Answer from the drawing. Dimensions are ordinates in mm from the lowest x, y and z of the part. A direction names the side the tool comes from. Round coordinates to 2 decimals unless told otherwise and drop trailing zeros. Loops run counter-clockwise (first coordinate to the right, second up) from the corner with the lowest first, then second, coordinate; pieces in that order, holes last. Notation, with made-up numbers: (86, 32.25) - (136, 32.25) arc R20 ccw to (136, 42.25) - close; hole circle Ø8 at (34.5, 70.5). An arc over 180 degrees is marked (long way). Write item = value, one per line. Start each with the question number.
1) A tool of negligible diameter and unlimited length cuts with its end or side. For the marked faces 4 and 5, from which of +Z, -Z, +X, -X, +Y, -Y can it reach the whole face along a straight path? Write none if from no direction.
2) Straight lines are drawn through the part: line 1 along X through (y, z) = (4, 5); line 2 along Y through (x, z) = (43, 18.75); line 3 along X through (y, z) = (6, 18). For each, find the intervals that lie inside material, in ascending order.
3) Section D-D, the plane y = 9.25 is taken. Determine the outline of the cut face in (x, z), and give its area (3 significant figures).
4) For a pull along X with two mould halves and no side action, classify the marked faces 1, 2 and 3 as released by +X, released by -X, zero draft, split by the parting line, or undercut.
5) Section B-B, the plane z = 15 is taken. Determine the outline of the cut face in (x, y), and give its area (3 significant figures).
6) Section C-C, the plane x = 23 is taken. Determine the outline of the cut face in (y, z), and give its area (3 significant figures).
7) Given pin 1 Ø2.5 at (x, z) = (44, 8) entering from -Y; pin 2 Ø4.5 at (y, z) = (7.5, 10) entering from -X; pin 3 Ø1.5 at (y, z) = (6.5, 17.5) entering from +X; pin 4 Ø8 at (x, y) = (14.5, 16) entering from -Z, each flat-ended and moving along its own axis, determine where each tip first touches the part or whether it passes through.
8) Section A-A, the plane y = 13.75 is taken. Determine the outline of the cut face in (x, z).
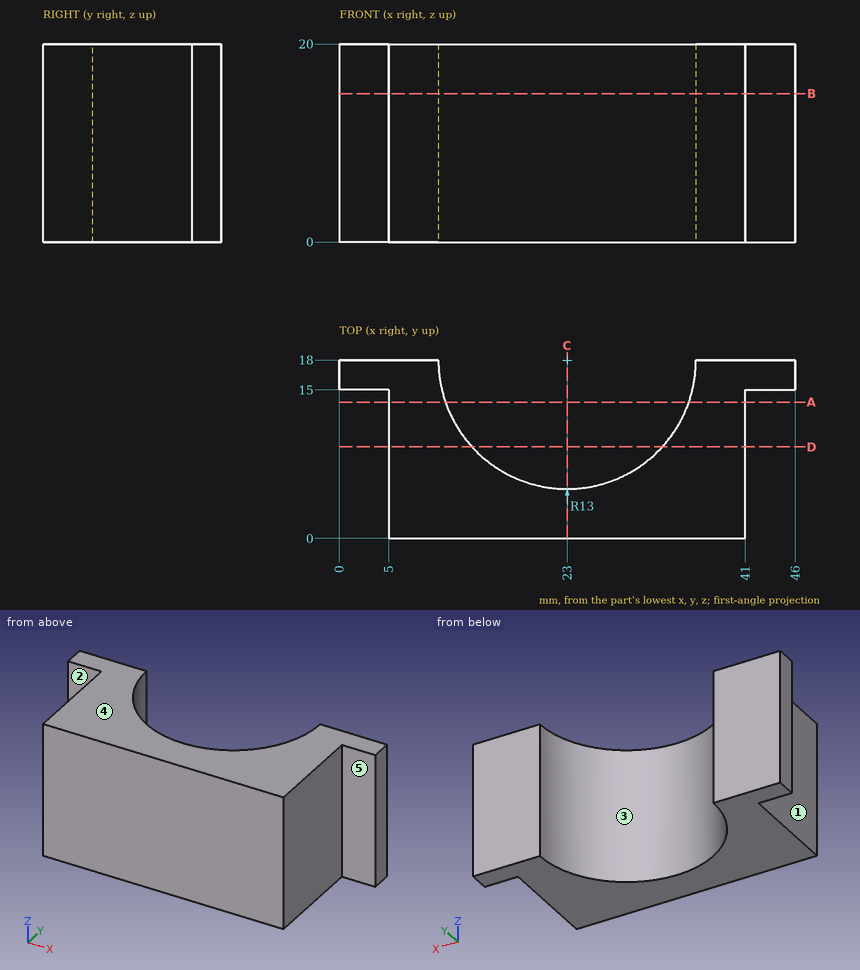
Geometry check:
q1.face_4 = +Z, +X, -X, +Y, -Y
q1.face_5 = +Z, -Z, +X, -Y
q2.line_1 = 5 to 41
q2.line_2 = 15 to 18
q2.line_3 = 5 to 18, 28 to 41
q3.outline = (5, 0) - (13.39, 0) - (13.39, 20) - (5, 20) - close; (32.61, 0) - (41, 0) - (41, 20) - (32.61, 20) - close
q3.area = 335 mm2
q4.face_1 = released by -X
q4.face_2 = zero draft
q4.face_3 = undercut
q5.outline = (0, 15) - (5, 15) - (5, 0) - (41, 0) - (41, 15) - (46, 15) - (46, 18) - (36, 18) arc R13 cw to (10, 18) - (0, 18) - close
q5.area = 413 mm2
q6.outline = (0, 0) - (5, 0) - (5, 20) - (0, 20) - close
q6.area = 100 mm2
q7.pin_1 = 15
q7.pin_2 = 5
q7.pin_3 = 41
q7.pin_4 = through
q8.outline = (5, 0) - (10.71, 0) - (10.71, 20) - (5, 20) - close; (35.29, 0) - (41, 0) - (41, 20) - (35.29, 20) - close
